Part model, mm, in its own coordinate system. A direction names the side the tool comes from. Coordinates: 2 decimals unless noted, no trailing zeros. Loops run counter-clockwise (first coordinate to the right, second up) from the corner with the lowest first, then second, coordinate; pieces in that order, holes last. Notation, with made-up numbers: (73, -19) - (129, -19) arc R14 ccw to (129, 1) - close; hole circle Ø3 at (-5, -39.5). An arc over 180 degrees is marked (long way). Use a Markdown table: item, result. Add a question column.
1) Band-saw the part on A-A (x = 0). Give the number of separate pieces and of enclosed holes in the cut face, plus the area to 3 significant figures.
2) Drop flat-ended pins along their axis: P1, Ø2.5, axis at x = -26.163, y = 26.163, coming from the +Z side; P2, Ø5, axis at y = -20.5, z = 10.5, coming from the +X side; P3, Ø4, axis at x = 19.5, z = 22, coming from the -Y side; P4, Ø1, axis at x = 0, z = 12.5, coming from the -Y side. Give the stop position or say it passes through.
3) Tool access for faces 1 (the face through (-16, -28, 23.5)), 2 (the face through (-41.965, -1.709, 20.965)), 3 (the face through (20.126, -6.338, 3.525)): list every direction of +Z, -Z, +X, -X, +Y, -Y with a clear straight run to the whole face (end or side of a thin tool).
4) Band-saw the part on C-C (z = 6). Give the cut face in (x, y), plus the area to 3 significant figures.
5) Probe probe 1 along Y at (x, z) = (0, 3); probe 2 along Y at (x, z) = (-1, 21.25); probe 3 along Z at (x, y) = (-34.5, 6.5). List the from-to ranges inside material, lowest first. Write a range as [from, to].
6) Pull direction X, two halves, no side cores. Call faces 4 (the face through (-6.94, 31.24, 9.12)), 5 (the face through (0, 22, 29)), 6 (the face through (-8, 16, 7.15)), 7 (the face through (38.5, -0.1, 21)): +X half, -X half, draft (parallel to the pull), parting line (faces both ways), or undercut.
7) Band-saw the part on D-D (y = -13). Give the cut face in (x, z), plus the area to 3 significant figures.
Solid Edge part; units mm, degrees
sketch "Sketch1" plane through (0, 0, 0) normal (0, 0, 1) x (1, 0, 0)
  circle A0 centre (0, 0) radius 32
  circle A1 centre (0, 0) radius 21.1
  circle A2 centre (27, 0) radius 1.7
  circle A3 centre (0, 27) radius 1.7
  circle A4 centre (-27, 0) radius 1.7
  circle A5 centre (0, -27) radius 1.7
extrude "Protrusion1" add sketch "Sketch1" along normal blind 7.15
sketch "Sketch2" plane through (0, 0, 7.15) normal (0, 0, 1) x (1, 0, 0)
  circle A0 centre (0, 0) radius 32
  circle A1 centre (0, 0) radius 17.5
  circle A2 centre (27, 0) radius 1.7
  circle A3 centre (0, 27) radius 1.7
  circle A4 centre (-27, 0) radius 1.7
  circle A5 centre (0, -27) radius 1.7
extrude "ExtrudedProtrusion_2" add sketch "Sketch2" along normal blind 14.7
sketch "Sketch3" plane through (0, 0, 21.85) normal (0, 0, 1) x (1, 0, 0)
  circle A0 centre (0, 0) radius 32
  circle A1 centre (0, 0) radius 21.1
  circle A2 centre (27, 0) radius 1.7
  circle A3 centre (0, 27) radius 1.7
  circle A4 centre (-27, 0) radius 1.7
  circle A5 centre (0, -27) radius 1.7
extrude "ExtrudedProtrusion_3" add sketch "Sketch3" along normal blind 7.15
sketch "Sketch4" plane through (0, 0, 18.5) normal (0, 0, 1) x (1, 0, 0)
  circle A0 centre (0, 0) radius 42
  circle A1 centre (0, 0) radius 17.5
  circle A2 centre (27, 0) radius 1.7
  circle A3 centre (0, 27) radius 1.7
  circle A4 centre (-27, 0) radius 1.7
  circle A5 centre (0, -27) radius 1.7
  circle A6 centre (26.163, 26.163) radius 1.7
  circle A7 centre (-26.163, 26.163) radius 1.7
  circle A8 centre (-26.163, -26.163) radius 1.7
  circle A9 centre (26.163, -26.163) radius 1.7
extrude "ExtrudedProtrusion_4" add sketch "Sketch4" along normal blind 5
sketch "Sketch5" plane through (0, 0, 21.85) normal (0, 0, 1) x (1, 0, 0)
  circle A0 centre (0, 0) radius 21.1
extrude "ExtrudedCutout_1" cut sketch "Sketch5" along normal blind 7.15
sketch "Sketch6" plane through (0, 0, 18.5) normal (0, 0, 1) x (1, 0, 0)
  circle A0 centre (60, 0) radius 21.5
extrude "ExtrudedCutout_2" cut sketch "Sketch6" along normal blind 5
Answer block:
| question | item | result |
|---|---|---|
| 1 | separate pieces | 4 |
| 1 | enclosed holes | 0 |
| 1 | area | 641 mm2 |
| 2 | P1 | through |
| 2 | P2 | x = 26.46 |
| 2 | P3 | y = -38.18 |
| 2 | P4 | y = -32 |
| 3 | face 1 | +Z |
| 3 | face 2 | +Z, -Z |
| 3 | face 3 | -Z |
| 4 | outline | circle Ø64 at (0, 0); hole circle Ø3.4 at (-27, 0); hole circle Ø42.2 at (0, 0); hole circle Ø3.4 at (0, -27); hole circle Ø3.4 at (0, 27); hole circle Ø3.4 at (27, 0) |
| 4 | area | 1,780 mm2 |
| 5 | probe 1 | [-32, -28.7], [-25.3, -21.1], [21.1, 25.3], [28.7, 32] |
| 5 | probe 2 | [-41.99, -28.37], [-25.63, -17.47], [17.47, 25.63], [28.37, 41.99] |
| 5 | probe 3 | [18.5, 23.5] |
| 6 | face 4 | parting line |
| 6 | face 5 | draft |
| 6 | face 6 | undercut |
| 6 | face 7 | +X half |
| 7 | outline | (-39.94, 18.5) - (-29.24, 18.5) - (-29.24, 0) - (-16.62, 0) - (-16.62, 7.15) - (-11.72, 7.15) - (-11.72, 21.85) - (-16.62, 21.85) - (-16.62, 29) - (-29.24, 29) - (-29.24, 23.5) - (-39.94, 23.5) - close; (11.72, 7.15) - (16.62, 7.15) - (16.62, 0) - (29.24, 0) - (29.24, 18.5) - (39.94, 18.5) - (39.94, 23.5) - (29.24, 23.5) - (29.24, 29) - (16.62, 29) - (16.62, 21.85) - (11.72, 21.85) - close |
| 7 | area | 983 mm2 |
